Source: CAD feature listing. Evaluate the final solid. Frame: model axes, mm. A direction names the side the tool comes from. Give positions to 0.01 mm unless a question says otherwise; leave off trailing zeros. Loops run counter-clockwise (first coordinate to the right, second up) from the corner with the lowest first, then second, coordinate; pieces in that order, holes last. Notation, with made-up numbers: M 8.25,36 L 55.25,36 A8 ccw 55.25,44 Z; hole C 74,53 d10. An arc over 180 degrees is marked long. Answer in a Markdown table with one row per item.
```python
from build123d import *

# Parameters (mm, degrees)
F0_R     = 6.35
F1_DEPTH = 38.1
F2_R     = 63.5
F3_DEPTH = 3.175
F4_W     = 6.35
F4_H     = 203.2
F4_W_2   = 203.2
F4_H_2   = 6.35
F5_DEPTH = 19.05
F6_R     = 63.5
F7_DEPTH = 3.175


with BuildPart() as f1:
    # F0 (on Top) → F1 (new body, symmetric)
    with BuildSketch(Plane.XY):
        Circle(F0_R)
    extrude(amount=F1_DEPTH, both=True)



with BuildPart() as f3:
    # F2 (on face) → F3 (new body)
    with BuildSketch(Plane.XY.offset(60.325)):
        Circle(F2_R)
    extrude(amount=F3_DEPTH)

    # F4 (on face) → F5 (join)
    with BuildSketch(Plane.XY.offset(41.275)):
        with Locations((0, 127)):
            Rectangle(F4_W, F4_H)
        with Locations((-127, 0)):
            Rectangle(F4_W_2, F4_H_2)
        with Locations((127, 0)):
            Rectangle(F4_W_2, F4_H_2)
        with Locations((0, -127)):
            Rectangle(F4_W, F4_H)
    extrude(amount=F5_DEPTH)


with BuildPart() as f1_1:
    add(f1.part)

    add(f3.part)  # F7 merges F3
    # F6 (on face) → F7 (join)
    with BuildSketch(Plane.XY.offset(38.1)):
        Circle(F6_R)
    extrude(amount=F7_DEPTH)


solid = f1_1.part
```
1) Section A-A, the plane z = 53.5. Return loops of the section in (x, y) (3 decimals), then the cut area to 3 significant figures.
Reply:
| item | result |
|---|---|
| outline | M -228.6,-3.175 L -25.4,-3.175 L -25.4,3.175 L -228.6,3.175 Z; M -3.175,-228.6 L 3.175,-228.6 L 3.175,-25.4 L -3.175,-25.4 Z; M -3.175,25.4 L 3.175,25.4 L 3.175,228.6 L -3.175,228.6 Z; M 25.4,-3.175 L 228.6,-3.175 L 228.6,3.175 L 25.4,3.175 Z |
| area | 5,160 mm² |
2) Pin query (flat end, axial travel): pin 1 Ø9.5 at (y, z) = (83, 48.5) entering from -X (3 decimals); pin 2 Ø9.5 at (x, z) = (152, 54.5) entering from +Y (3 decimals); pin 3 Ø5 at (x, y) = (145, -0.5) entering from +Z (3 decimals). Return the tip coordinate at first contact, or that it passes through.
Reply:
| item | result |
|---|---|
| pin 1 | stops at x = -3.175 |
| pin 2 | stops at y = 3.175 |
| pin 3 | stops at z = 60.325 |
3) Material intervals for L1, parallel to X at y = -111.5, z = 50 (3 decimals), sorted ascending.
Reply:
| item | result |
|---|---|
| L1 | x = -3.175 to 3.175 |
4) Pull-direction query (Z, two-part tool) for faces 1 (the flat face through (13, 1, 38.1)), 2 (the flat face through (126, 3.175, 51)), 3 (the flat face through (-1, 1, 63.5)); classes: released by +Z, released by -Z, zero draft, split by the parting line, or undercut.
Reply:
| item | result |
|---|---|
| face 1 | released by -Z |
| face 2 | undercut |
| face 3 | released by +Z |
5) Section B-B, the plane y = -161.5. Return loops of the section in (x, z) (3 decimals), then the cut area to 3 significant figures.
Reply:
| item | result |
|---|---|
| outline | M -3.175,41.275 L 3.175,41.275 L 3.175,60.325 L -3.175,60.325 Z |
| area | 121 mm² |
6) Set-up query: faces 4 (the flat face through (-3.175, 126, 51)), 5 (the flat face through (-128, 3.175, 51)), 6 (the flat face through (-1, 1, 41.275)), 7 (the flat face through (126, -3.175, 51)), 8 (the flat face through (3.175, -128, 51)). Return all of +Z, -Z, +X, -X, +Y, -Y with unobstructed straight access to the full face (end or side cutting, diameter ignored); none if empty.
Reply:
| item | result |
|---|---|
| face 4 | -X, +Y, -Y |
| face 5 | +X, -X, +Y |
| face 6 | none |
| face 7 | +X, -X, -Y |
| face 8 | +X, +Y, -Y |
